Input: part model. Units: mm. Frame: model coordinates. A direction names the side the tool comes from. Round coordinates to 2 decimals unless told otherwise and drop trailing zeros. Order: outer loops, then holes, each group sorted by start corner. A loop starts at its lowest first (then second) coordinate and runs counter-clockwise, first axis right, second up.
Item 1: Mould query, pull axis X, two halves, no side actions, for faces 4 (the conical face through (4.64, -0.06, -3.14)), 5 (the cylindrical face through (0.135, -2.252, 6.274)), 6 (the flat face through (0, 6.25, 0)). Classes: released by +X, released by -X, zero draft, split by the parting line, or undercut.
Item 2: Cut plane B-B on x = 2.75. Output: boundary loops of the cut face in (y, z).
Item 3: Line query: L1, parallel to Z at x = -2.5, y = 0; L2, parallel to Y at x = 0.5, z = 2; L3, parallel to Y at x = 0, z = -2.75. Output: solid intervals per line, ascending.
Item 4: Cut plane A-A on y = 0. Give the number of separate pieces and of enclosed holes in the cut face, then the cut area to 3 significant figures.
Item 5: Reachability of faces 1 (the conical face through (-4.64, 0.06, -3.14)), 2 (the flat face through (0, 5, -0.5)), 3 (the flat face through (2, -4, 4)) from +Z, -Z, +X, -X, +Y, -Y: full face, straight path, thin tool, end or side. Return the list, or none.
Item 6: First-contact query: pin 1 (4 mm diameter, centred on x = 0, y = -6, fed in from -Z); pin 2 (1 mm diameter, centred on x = -0.5, y = 2, fed in from +Z); pin 3 (2 mm diameter, centred on y = 0, z = 6.5, fed in from +X); pin 4 (1.5 mm diameter, centred on y = -1, z = -6.5, fed in from -X). Flat tips, straight axial feed; report the tip coordinate or a pass-through.
Autodesk Inventor part; units mm, degrees
ref_plane "body_screw_XY" through (0, -6, 4) normal (0, 0, 1) x (1, 0, 0)
ref_plane "body_screw_YZ" through (0, -6, 4) normal (1, 0, 0) x (0, 1, 0)
ref_plane "body_screw_ZX" through (0, -6, 4) normal (0, 1, 0) x (0, 0, 1)
sketch "Sketch_1" plane through (0, 0, 0) normal (0, 0, 1) x (1, 0, 0)
  line L0 (5, 0) -> (-5, 0)
  line L1 (-5, 9.5) -> (-5, 3.5)
  line L2 (-5, 3.5) -> (-4.5, 3)
  line L3 (-4.5, 3) -> (4.5, 3)
  line L4 (4.5, 3) -> (5, 3.5)
  line L5 (5, 3.5) -> (5, 9.5)
  line L6 (5, 9.5) -> (4.5, 10)
  line L7 (4.5, 10) -> (-4.5, 10)
  line L8 (-4.5, 10) -> (-5, 9.5)
revolve "Revolution1" add sketch "Sketch_1" angle 360 about axis through (5, 0, 0) along (1, 0, 0)
sketch "Sketch_2" plane through (0, 0, 0) normal (1, 0, 0) x (0, 1, 0)
  line L0 (-10, 0.5) -> (-10, -0.5)
  line L1 (-10, -0.5) -> (6.25, -0.5)
  line L2 (6.25, -0.5) -> (6.25, 0.5)
  line L3 (6.25, 0.5) -> (-10, 0.5)
extrude "Extrusion1" cut sketch "Sketch_2" along normal mid plane 10
sketch "Sketch_3" plane through (0, 0, 0) normal (1, 0, 0) x (0, 1, 0)
  line L0 (-6, 10) -> (-6, 0)
  line L1 (-6, 0) -> (-8.25, 0)
  line L2 (-8.25, 0) -> (-8.25, 4)
  line L3 (-8.25, 4) -> (-9.75, 4)
  line L4 (-9.75, 4) -> (-9.75, 10)
  line L5 (-9.75, 10) -> (-6, 10)
  line L6 (-6, 10) -> (-6, 0)
revolve "Revolution2" cut sketch "Sketch_3" angle 360 about axis through (0, -6, 10) along (0, 0, 1)
sketch "Sketch_4" plane through (0, 0, 0) normal (1, 0, 0) x (0, 1, 0)
  line L0 (-6, -9.5) -> (-6, -0.5)
  line L1 (-6, -0.5) -> (-4, -0.5)
  line L2 (-4, -0.5) -> (-4.379, -0.879)
  line L3 (-4.379, -0.879) -> (-4.379, -9.5)
  line L4 (-4.379, -9.5) -> (-6, -9.5)
  line L5 (-6, -9.5) -> (-6, -0.5)
revolve "Revolution3" cut sketch "Sketch_4" angle 360 about axis through (0, -6, -9.5) along (0, 0, -1)
thread "Thread1"
sketch "Sketch_7" plane through (0, 0, -6.5) normal (0, 0, 1) x (1, 0, 0)
  line L0 (5, 0) -> (-5, 0)
  line L1 (-5, 0) -> (-5, 1.5)
  line L2 (-5, 1.5) -> (-4.7295, 1.2295)
  line L3 (-4.7295, 1.2295) -> (4.7295, 1.2295)
  line L4 (4.7295, 1.2295) -> (5, 1.5)
  line L5 (5, 1.5) -> (5, 0)
  line L6 (5, 0) -> (-5, 0)
revolve "Revolution4" cut sketch "Sketch_7" angle 360 about axis through (5, 0, -6.5) along (1, 0, 0)
thread "Thread2"
sketch "Sketch_8" plane through (0, 0, 6.5) normal (0, 0, 1) x (1, 0, 0)
  line L0 (5, 0) -> (-5, 0)
  line L1 (-5, 0) -> (-5, 1.5)
  line L2 (-5, 1.5) -> (-4.7295, 1.2295)
  line L3 (-4.7295, 1.2295) -> (4.7295, 1.2295)
  line L4 (4.7295, 1.2295) -> (5, 1.5)
  line L5 (5, 1.5) -> (5, 0)
  line L6 (5, 0) -> (-5, 0)
revolve "Revolution5" cut sketch "Sketch_8" angle 360 about axis through (5, 0, 6.5) along (1, 0, 0)
thread "Thread3"
ref_plane "body_screw_XY" through (0, -6, 4) normal (0, 0, 1) x (1, 0, 0)
ref_plane "body_screw_YZ" through (0, -6, 4) normal (1, 0, 0) x (0, 1, 0)
ref_plane "body_screw_ZX" through (0, -6, 4) normal (0, 1, 0) x (0, 0, 1)
properties part number "SCSW6-10b"
From the geometry:
1. face 4: released by +X
1. face 5: undercut
1. face 6: zero draft
2. outline: (-9.99, -0.5) arc R10 ccw (long way) to (-3.45, 9.39) - (-3.45, 4) - (-8.55, 4) - (-8.55, 5.19) arc R10 ccw to (-9.99, 0.5) - (-2.96, 0.5) arc R3 cw to (2.96, 0.5) - (6.25, 0.5) - (6.25, -0.5) - (2.96, -0.5) arc R3 cw to (-2.96, -0.5) - close; hole circle Ø2.46 at (0, -6.5); hole circle Ø2.46 at (0, 6.5)
3. L1: z = -10 to -7.73, -5.27 to -3, 3 to 5.27, 7.73 to 10
3. L2: y = -9.8 to -8.19, -3.81 to -2.24, 2.24 to 9.8
3. L3: y = -9.61 to -7.62, -4.38 to -1.2, 1.2 to 9.61
4. separate pieces: 4
4. enclosed holes: 0
4. area: 89.5 mm2
5. face 1: -X
5. face 2: +X, -X, -Y
5. face 3: +Z
6. pin 1: stops at z = -9.17
6. pin 2: stops at z = 9.89
6. pin 3: passes through
6. pin 4: stops at x = -5
